Geometry: final body of the model. Coordinates: model frame, mm. Round coordinates to 2 decimals unless told otherwise and drop trailing zeros. Order: outer loops, then holes, each group sorted by start corner. A loop starts at its lowest first (then second) coordinate and runs counter-clockwise, first axis right, second up. Notation, with made-up numbers: M -29.5,50 L -5.5,50 A8 cw -5.5,60 Z; hole C -19.75,23 d7. An arc over 180 degrees is marked long. Return JSON: item names as keys, results as strings. Group by question number.
Q1. Cut plane B-B on z = -67.5. Output: boundary loops of the cut face in (x, y), and give its area (3 significant figures).
Q2. Ray query, probe 1 along Z at (x, y) = (228.6, 2); probe 2 along Z at (x, y) = (314.5, 4.5); probe 3 along X at (y, z) = (0.75, -86.5). Return the intervals inside material, ascending.
Q3. Contact query for flat-ended pins moving along their axis: pin 1 (7.5 mm diameter, centred on x = 143.93, z = -141.2, fed in from -Y); pin 2 (21.5 mm diameter, centred on x = 228.6, z = -75.56, fed in from -Y). Output: stop coordinate, or through.
Q4. Cut plane C-C on y = 4.5. Output: boundary loops of the cut face in (x, z), and give its area (3 significant figures).
Q5. Cut plane A-A on x = 228.6. Output: boundary loops of the cut face in (y, z).
Q6. Mould query, pull axis X, two halves, no side actions, for faces 1 (the face through (146.77, 3.13, -66.01)), 2 (the face through (230, 0, -100)), 3 (the face through (330.2, 3, -102)). Classes: released by +X, released by -X, zero draft, split by the parting line, or undercut.
Autodesk Inventor part; units mm, degrees
ref_plane "YZ Plane" through (0, 0, 0) normal (1, 0, 0) x (0, 1, 0)
ref_plane "XZ Plane" through (0, 0, 0) normal (0, 1, 0) x (-1, 0, 0)
ref_plane "XY Plane" through (0, 0, 0) normal (0, 0, 1) x (1, 0, 0)
sketch "Sketch1" plane through (0, 0, 0) normal (0, 1, 0) x (-1, 0, 0)
  line L0 (-330.2, -201.9268) -> (-330.2, 0)
  line L1 (-127, -201.9268) -> (-330.2, -201.9268)
  line L2 (-330.2, 0) -> (-127, 0)
  line L3 (-127, 0) -> (-127, -201.9268)
  point P0 (0, 0)
  dimension "d136" = 203.2
extrude "Extrusion1" add sketch "Sketch1" along normal blind 6.35
sketch "Sketch2" plane through (0, 6.35, 0) normal (0, 1, 0) x (1, 0, 0)
  circle A0 centre (143.9333, 141.1986) radius 2.6501
  circle A1 centre (143.9333, 67.4878) radius 2.6501
  circle A2 centre (313.2667, 141.1986) radius 2.6501
  circle A3 centre (313.2667, 67.4878) radius 2.6501
  line L0 (330.2, 0) -> (127, 0)
  line L1 (127, 0) -> (330.2, 0)
  line L2 (330.2, 0) -> (330.2, 201.9268)
  line L3 (330.2, 0) -> (330.2, 201.9268)
  line L4 (330.2, 201.9268) -> (127, 201.9268)
  line L5 (127, 201.9268) -> (127, 0)
  line L6 (127, 201.9268) -> (127, 0)
  point P0 (127, 19.4733)
  point P1 (330.2, 149.86)
  point P2 (228.6, 0)
  dimension "d137" = 203.2
hole "Hole9" at (143.9333, 6.35, -141.1986) direction (0, -1, 0) diameter 6.4008 end through all
hole "Hole10" at (143.9333, 6.35, -67.4878) direction (0, -1, 0) diameter 6.4008 end through all
hole "Hole11" at (313.2667, 6.35, -141.1986) direction (0, -1, 0) diameter 6.4008 end through all
hole "Hole12" at (313.2667, 6.35, -67.4878) direction (0, -1, 0) diameter 6.4008 end through all
sketch "Sketch3" plane through (0, 6.35, 0) normal (0, 1, 0) x (1, 0, 0)
  circle A0 centre (228.6, 75.5634) radius 17.9959
  point P0 (0, 0)
  point P1 (127, 201.9268)
extrude "Extrusion2" cut sketch "Sketch3" against normal blind 50.8
equation "\"d97\" = d12"
equation "\"d104\" = d12"
equation "\"d111\" = d12"
properties part number "base_plate"
Result sheet:
{
 "1": {"outline": "M 127,0 L 140.73,0 L 140.73,6.35 L 127,6.35 Z; M 147.13,0 L 212.51,0 L 212.51,6.35 L 147.13,6.35 Z; M 244.69,0 L 310.07,0 L 310.07,6.35 L 244.69,6.35 Z; M 316.47,0 L 330.2,0 L 330.2,6.35 L 316.47,6.35 Z", "area": "1,000 mm²"},
 "2": {"probe 1": "z = -201.93 to -93.56, -57.57 to 0", "probe 2": "z = -201.93 to -144.15, -138.25 to -70.44, -64.53 to 0", "probe 3": "x = 127 to 214.31, 242.89 to 330.2"},
 "3": {"pin 1": "stops at y = 0", "pin 2": "passes through"},
 "4": {"outline": "M 127,-201.93 L 330.2,-201.93 L 330.2,0 L 127,0 Z; hole C 143.93,-141.2 d6.4; hole C 143.93,-67.49 d6.4; hole C 228.6,-75.56 d35.99; hole C 313.27,-141.2 d6.4; hole C 313.27,-67.49 d6.4", "area": "39,900 mm²"},
 "5": {"outline": "M 0,-201.93 L 6.35,-201.93 L 6.35,-93.56 L 0,-93.56 Z; M 0,-57.57 L 6.35,-57.57 L 6.35,0 L 0,0 Z"},
 "6": {"face 1": "undercut", "face 2": "zero draft", "face 3": "released by +X"}
}
